```python
from build123d import *

# Parameters (mm, degrees)
BOSS_EXTRUDE2_DEPTH = 50
SKETCH2_R           = 27.5
BOSS_EXTRUDE3_DEPTH = 150
BOSS_EXTRUDE4_START = -150
BOSS_EXTRUDE4_DEPTH = 150


with BuildPart() as part:
    # Sketch1 → Boss-Extrude2 (new body)
    with BuildSketch(Plane.XY):
        Polygon((-500, 250), (500, 250), (500, 200), (450, 200), (450, 50), (500, 50), (500, 0), (-500, 0), (-500, 50), (-450, 50), (-450, 200), (-500, 200), align=None)
    extrude(amount=BOSS_EXTRUDE2_DEPTH)

    # Sketch2 → Boss-Extrude3 (add)
    with BuildSketch(Plane.XZ.offset(-200)):
        with Locations(Location((-490, 25, 0), (0, 0, 65.380022671))):
            Circle(SKETCH2_R)
    boss_extrude3 = extrude(amount=BOSS_EXTRUDE3_DEPTH)

    # Mirror1: Boss-Extrude3 across plane
    add(boss_extrude3.mirror(Plane(origin=(0, 0, 0), x_dir=(0, 0, 1), z_dir=(1, 0, 0))))

    # Sketch3 → Boss-Extrude4 (add)
    with BuildSketch(Plane.XZ.offset(-50).offset(BOSS_EXTRUDE4_START)):
        with BuildLine():
            Line((-490, 54.5), (490, 54.5))
            ThreePointArc((490, 54.5), (519.5, 25), (490, -4.5))
            Line((490, -4.5), (-490, -4.5))
            ThreePointArc((-490, -4.5), (-519.5, 25), (-490, 54.5))
        make_face()
        with BuildLine():
            Line((-490, 52.5), (490, 52.5))
            ThreePointArc((490, 52.5), (517.5, 25), (490, -2.5))
            Line((490, -2.5), (-490, -2.5))
            ThreePointArc((-490, -2.5), (-517.5, 25), (-490, 52.5))
        make_face(mode=Mode.SUBTRACT)
    extrude(amount=BOSS_EXTRUDE4_DEPTH)


solid = part.part
```
Model file for the job. Use its own axes, mm. A direction names the side the tool comes from. Coordinates: 2 decimals unless noted, no trailing zeros. Write each loop counter-clockwise with the first axis right and the second up, starting at its lowest first coordinate (ties: lowest second). Pieces come first, ordered by that corner, then holes. Notation, with made-up numbers: (-23, 18.5) - (2, 18.5) arc R22 ccw to (2, 31.5) - close; hole circle Ø6 at (-39.75, 1). An arc over 180 degrees is marked (long way). One line per question, with ' | ' between items. Start each with the question number.
Q1. 3-axis set-ups, long thin cutter, end or side, ignore diameter. For faces 1 (the face through (-458, 50, 25)), 2 (the face through (-500, 225, 25)), 3 (the face through (-7, 126, 52.5)), 4 (the face through (500, 225, 25)): which of +Z, -Z, +X, -X, +Y, -Y reach the whole face in a straight line?
Q2. Cut at A-A, the plane y = 188. List the corners of the cut face in (x, z), then the cut area to 3 significant figures.
Q3. Pin check, flat tips, straight feed: pin 1 (5 mm diameter, centred on y = 171.5, z = 38.5, fed in from -X); pin 2 (25 mm diameter, centred on y = 16, z = 35, fed in from -X); pin 3 (25 mm diameter, centred on y = 131, z = 14, fed in from -X). Stop position of each tip, or through.
Q4. Cut at B-B, the plane x = 101.5. List the corners of the cut face in (y, z), then the cut area to 3 significant figures.
Q5. Pull direction Y, two halves, no side cores. Call faces 5 (the face through (7, 0, 25)), 6 (the face through (458, 50, 25)), 7 (the face through (-500, 25, 25)): pulls with the +Y half, pulls with the -Y half, needs draft (parallel to the pull), parting line crosses it, or undercut.
Q6. Drill centre lines: line 1 (Z direction, x = -13, y = 153); line 2 (X direction, y = 144, z = 22); line 3 (X direction, y = 86.5, z = 23). Where is each one in solid material? Low to high. Write a range as [from, to].
Answer below:
1) face 1: none | face 2: +Z, -Z, -X, +Y | face 3: +Y, -Y | face 4: +Z, -Z, +X, +Y
2) outline: (-490, -4.5) - (490, -4.5) arc R29.5 ccw to (490, 54.5) - (-490, 54.5) arc R29.5 ccw to start; (-450, 0) - (450, 0) - (450, 50) - (-450, 50) - close; hole (-490, -2.5) - (490, -2.5) arc R27.5 cw to (490, 52.5) - (-490, 52.5) arc R27.5 cw to start | area: 54,000 mm^2
3) pin 1: x = -517.37 | pin 2: x = -500 | pin 3: x = -519.5
4) outline: (0, 0) - (250, 0) - (250, 50) - (0, 50) - close; (50, -4.5) - (200, -4.5) - (200, -2.5) - (50, -2.5) - close; (50, 52.5) - (200, 52.5) - (200, 54.5) - (50, 54.5) - close | area: 13,100 mm^2
5) face 5: pulls with the -Y half | face 6: undercut | face 7: needs draft
6) line 1: [-4.5, -2.5], [0, 50], [52.5, 54.5] | line 2: [-519.35, -462.66], [-450, 450], [462.66, 519.35] | line 3: [-519.43, -462.57], [-450, 450], [462.57, 519.43]
